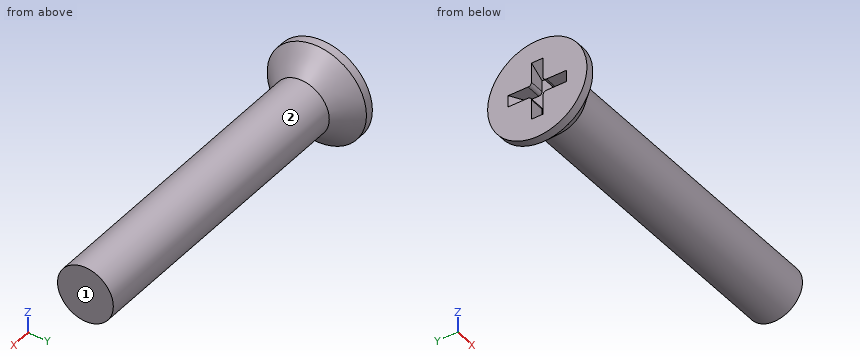
from build123d import *

# Parameters (mm, degrees)
CROSSRECESS_DEPTH = 1.35
DRAFT9_ANGLE      = 30
FILLET5_R         = 0.3
SKETCH10_W        = 0.8
SKETCH10_H        = 2.5


with BuildPart() as part:
    # Sketch1 → Base (revolve)
    with BuildSketch(Plane.XY):
        Polygon((30, 2.5), (4.3, 2.5), (2.7, 2.5), (0.75, 4.45), (0, 4.45), (0, 0), (30, 0), align=None)
    revolve(axis=Axis((4.515812911, 0, 0), (-1, 0, 0)))

    # Sketch6 → CrossRecess (cut)
    with BuildSketch(Plane(origin=(0, 0, 0), x_dir=(0, 0, -1), z_dir=(1, 0, 0))):
        Polygon((0.52, 0.52), (0.52, 2.6), (-0.52, 2.6), (-0.52, 0.52), (-2.6, 0.52), (-2.6, -0.52), (-0.52, -0.52), (-0.52, -2.6), (0.52, -2.6), (0.52, -0.52), (2.6, -0.52), (2.6, 0.52), align=None)
    extrude(amount=CROSSRECESS_DEPTH, mode=Mode.SUBTRACT)

    # Draft9
    draft9_faces = [part.faces().sort_by_distance(p)[0] for p in [
        (0.675, -2.6, 0),
        (0.675, 0, 2.6),
        (0.675, 0, -2.6),
        (0.675, 2.6, 0),
    ]]
    draft(draft9_faces, Plane(origin=(0, 4.45, 0), x_dir=(0, 0, -1), z_dir=(-1, 0, 0)), DRAFT9_ANGLE)

    # Fillet5
    fillet5_edges = [part.edges().sort_by_distance(p)[0] for p in [
        (0.675, 0.52, 0.52),
        (0.675, -0.52, 0.52),
        (0.675, -0.52, -0.52),
        (0.675, 0.52, -0.52),
    ]]
    fillet(fillet5_edges, radius=FILLET5_R)

    # Sketch10 → Revolve2 (revolve)
    with BuildSketch(Plane.XY):
        with Locations((3.1, 1.25)):
            Rectangle(SKETCH10_W, SKETCH10_H)
    revolve(axis=Axis((62.228915663, 0, 0), (-1, 0, 0)))


solid = part.part
Design review of the part built by this model. Coordinates are the model's own, in mm. Face numbers are marked on the shaded views. A direction names the side the tool comes from. Round coordinates to 2 decimals unless told otherwise and drop trailing zeros. Loops run counter-clockwise (first coordinate to the right, second up) from the corner with the lowest first, then second, coordinate; pieces in that order, holes last. Notation, with made-up numbers: (10.25, 76.5) - (47.25, 76.5) arc R25 ccw to (47.25, 102.5) - close; hole circle Ø6 at (16, -2). An arc over 180 degrees is marked (long way). One line per item, written item: value. Start each with the question number.
1) Insertion check: pin 1 Ø0.7 at (x, y) = (0.5, -1.5) entering from -Z; pin 2 Ø0.7 at (x, z) = (0.5, 1.5) entering from -Y; pin 3 Ø4 at (x, y) = (17.5, -0.5) entering from +Z. Each pin has a flat end and moves straight along its axis. Give the tip position at first contact, or say it passes through.
2) To check wall thickness, follow L1, parallel to Y at x = 19.75, z = 0; L2, parallel to X at y = 3.25, z = 2.25; L3, parallel to X at y = 0.25, z = -0.5. State the ranges of each line that lie inside material, in increasing order. Write a range as from..to.
3) For the marked faces 1 and 2, list the 3-axis set-ups (+Z, -Z, +X, -X, +Y, -Y) from which the entire face can be reached by the end or side of a thin tool; tool diameter is ignored.
4) Consider section A-A on z = 0. Give the boundary of the cut face in (x, y), then the cut area to 3 significant figures.
5) Consider section C-C on x = 18.75. Give the boundary of the cut face in (y, z), then the cut area to 3 significant figures.
Reported:
1. pin 1: stops at z = -4.3
1. pin 2: stops at y = -4.3
1. pin 3: stops at z = 2.5
2. L1: y = -2.5..2.5
2. L2: x = 0..1.25
2. L3: x = 1.35..30
3. face 1: +Z, -Z, +X, +Y, -Y
3. face 2: +X
4. outline: (0, -4.45) - (0.75, -4.45) - (2.7, -2.5) - (30, -2.5) - (30, 2.5) - (2.7, 2.5) - (0.75, 4.45) - (0, 4.45) - (0, 2.6) - (1.35, 1.82) - (1.35, -1.82) - (0, -2.6) - close
4. area: 151 mm^2
5. outline: circle Ø5 at (0, 0)
5. area: 19.6 mm^2
